Here's how the part is built. I have some questions about the finished solid (model axes, mm). A direction names the side the tool comes from. Round coordinates to 2 decimals unless told otherwise and drop trailing zeros. Write each loop counter-clockwise with the first axis right and the second up, starting at its lowest first coordinate (ties: lowest second). Pieces come first, ordered by that corner, then holes. Notation, with made-up numbers: (-8.75, 19.25) -> (13.25, 19.25) arc R26 cw to (13.25, 45.25) -> close; hole circle Ø6 at (24, 24.5). An arc over 180 degrees is marked (long way). Answer in a Markdown table with one row per item.
from build123d import *

# Parameters (mm, degrees)
CHAMFER1_SIZE = 1.27


with BuildPart() as part:
    # Sketch1 → Shaft (revolve)
    with BuildSketch(Plane.XY, mode=Mode.PRIVATE) as shaft_sk:
        Polygon((0, 0), (114.3, 0), (114.3, 6.35), (88.9, 6.35), (88.9, 9.525), (38.1, 9.525), (38.1, 12.7), (0, 12.7), align=None)
    revolve(shaft_sk.sketch.rotate(Axis((0, 0, 0), (1, 0, 0)), 90), axis=Axis((0, 0, 0), (1, 0, 0)))

    # Chamfer1
    chamfer1_edges = [part.edges().sort_by_distance(p)[0] for p in [
        (0, 0, -12.7),
        (114.3, 0, -6.35),
    ]]
    chamfer(chamfer1_edges, length=CHAMFER1_SIZE)


solid = part.part
1) Which directions (+Z, -Z, +X, -X, +Y, -Y) give clear straight access to the entire face, cutting with the end or side of a thin tool? Please do faces 1 (the face through (0, 0, 0)), 2 (the face through (100.8, 3.86, -5.04)).
Response:
| item | result |
|---|---|
| face 1 | +Z, -Z, -X, +Y, -Y |
| face 2 | +X |
2) I want a section at C-C, the plane x = 66.5. List the corners of the cut face in (y, z) for me (3 decimals), and give its area (3 significant figures).
Response:
| item | result |
|---|---|
| outline | circle Ø19.05 at (0, 0) |
| area | 285 mm^2 |
3) For pin 1 (10 mm diameter, centred on x = 57.5, z = 0, fed in from +Y) (3 decimals); pin 2 (8 mm diameter, centred on x = 54.5, y = -7.5, fed in from +Z); pin 3 (1 mm diameter, centred on x = 63, y = -4.5, fed in from -Z), each with a flat end and sliding along its axis, tell me the tip position at first contact or that it passes through.
Response:
| item | result |
|---|---|
| pin 1 | stops at y = 9.525 |
| pin 2 | stops at z = 8.86 |
| pin 3 | stops at z = -8.64 |
4) I need wall thicknesses on line 1 (Y direction, x = 88.5, z = 0.5); line 2 (Y direction, x = 34.5, z = -11); line 3 (X direction, y = 9.5, z = -1.25). Which ranges of each line are inside material? Lowest first, please. Write a range as [from, to].
Response:
| item | result |
|---|---|
| line 1 | y = [-9.51, 9.51] |
| line 2 | y = [-6.35, 6.35] |
| line 3 | x = [0, 38.1] |
5) I want a section at A-A, the plane y = 0. List the corners of the cut face in (x, z) for me (3 decimals), and give its area (3 significant figures).
Response:
| item | result |
|---|---|
| outline | (0, -11.43) -> (1.27, -12.7) -> (38.1, -12.7) -> (38.1, -9.525) -> (88.9, -9.525) -> (88.9, -6.35) -> (113.03, -6.35) -> (114.3, -5.08) -> (114.3, 5.08) -> (113.03, 6.35) -> (88.9, 6.35) -> (88.9, 9.525) -> (38.1, 9.525) -> (38.1, 12.7) -> (1.27, 12.7) -> (0, 11.43) -> close |
| area | 2,250 mm^2 |
